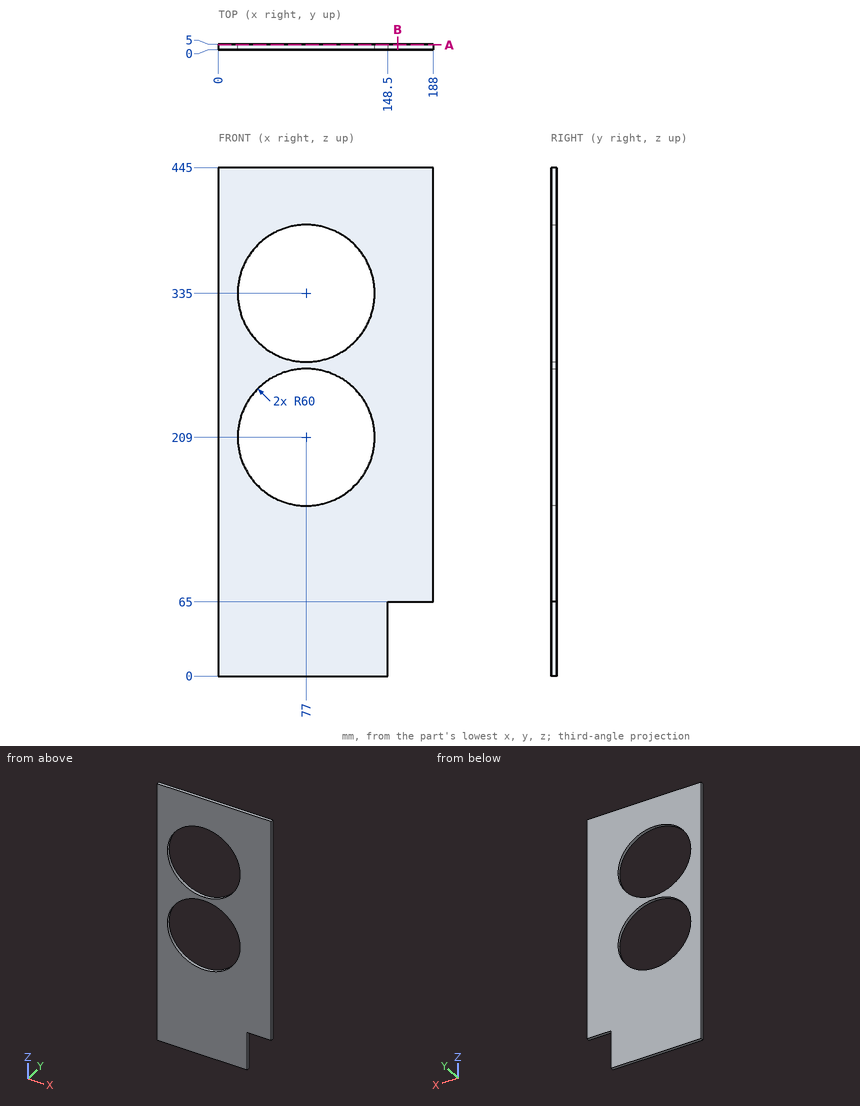
Input: dimensioned drawing with shaded views. Units: mm. Origin: part minimum x, y, z. Coordinates: 2 decimals unless noted, no trailing zeros. Loops run counter-clockwise (first coordinate to the right, second up) from the corner with the lowest first, then second, coordinate; pieces in that order, holes last. Notation, with made-up numbers: M -3,28.25 L 30,28.25 A20 ccw 30,66.25 Z; hole C 64,62.5 d4. An arc over 180 degrees is marked long. Put each result on its own line as item: value.
(1) Cut plane B-B on x = 157. Return the cut outline in (y, z).
Answer sheet:
outline: M 0,65 L 5,65 L 5,445 L 0,445 Z
(2) Cut plane A-A on y = 4.2. Return the cut outline in (x, z).
Answer sheet:
outline: M 0,0 L 148.5,0 L 148.5,65 L 188,65 L 188,445 L 0,445 Z; hole M 17,209 A60 ccw long 77,269 A60 ccw Z; hole C 77,335 d120
(3) Material intervals for probe 1 along Z at (x, y) = (77, 1.3); probe 2 along Z at (x, y) = (41, 0.85); probe 3 along X at (y, z) = (3.25, 335.5), sorted ascending.
Answer sheet:
probe 1: z = 0 to 149, 269 to 275, 395 to 445
probe 2: z = 0 to 161, 257 to 287, 383 to 445
probe 3: x = 0 to 17, 137 to 188
(4) First-contact query: pin 1 (1.5 mm diameter, centred on y = 3.5, z = 364, fed in from -X); pin 2 (1.5 mm diameter, centred on x = 160.5, y = 3.5, fed in from -Z). Flat tips, straight axial feed; report the tip coordinate or a pass-through.
Answer sheet:
pin 1: stops at x = 0
pin 2: stops at z = 65
